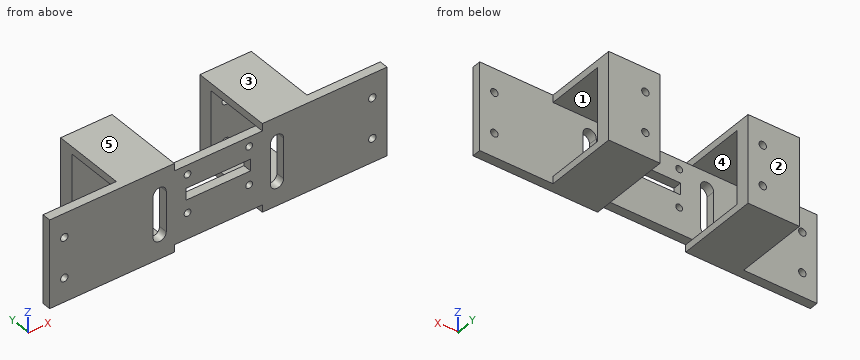
```python
from build123d import *

# Parameters (mm, degrees)
SKETCH1_W                         = 30
SKETCH1_H                         = 25
SKETCH1_R                         = 1.15
SKETCH1_W_2                       = 22
SKETCH1_H_2                       = 4
BOSS_EXTRUDE1_DEPTH               = 3
SKETCH2_W                         = 7.5
SKETCH2_H                         = 20
SKETCH2_R                         = 1.27
BOSS_EXTRUDE2_DEPTH               = 3
SKETCH6_W                         = 20
SKETCH6_H                         = 3
BOSS_EXTRUDE3_DEPTH               = 10
SKETCH7_W                         = 20
SKETCH7_H                         = 3
BOSS_EXTRUDE4_DEPTH               = 10
SKETCH8_W                         = 17.5
SKETCH8_H                         = 20
SKETCH8_R                         = 1.27
BOSS_EXTRUDE5_DEPTH               = 25
SKETCH13_W                        = 17.5
SKETCH13_H                        = 28
BOSS_EXTRUDE6_DEPTH               = 5
SKETCH14_W                        = 17.5
SKETCH14_H                        = 28
BOSS_EXTRUDE7_DEPTH               = 5
SKETCH15_W                        = 25
SKETCH15_H                        = 20
CUT_EXTRUDE2_DEPTH                = 48.5
CUT_EXTRUDE2_DEPTH_BACK           = 18.5
SKETCH16_W                        = 30
SKETCH16_H                        = 3
BOSS_EXTRUDE8_DEPTH               = 25
SKETCH19_W                        = 30
SKETCH19_H                        = 3
BOSS_EXTRUDE9_DEPTH               = 25
F_1_16_0_0625_PRESS_DOWEL_HOLE1_D = 2.54
CUT_EXTRUDE3_DEPTH                = 4


with BuildPart() as part:
    # Sketch1 → Boss-Extrude1 (new body)
    with BuildSketch(Plane(origin=(0, 0, 0), x_dir=(1, 0, 0), z_dir=(0, 1, 0))):
        with Locations((-15, 0)):
            Rectangle(SKETCH1_W, SKETCH1_H)
        with Locations((-4.5, 3.7)):
            Circle(SKETCH1_R, mode=Mode.SUBTRACT)
        with Locations((-4.5, -9.3)):
            Circle(SKETCH1_R, mode=Mode.SUBTRACT)
        with Locations((-25.5, 3.7)):
            Circle(SKETCH1_R, mode=Mode.SUBTRACT)
        with Locations((-25.5, -9.3)):
            Circle(SKETCH1_R, mode=Mode.SUBTRACT)
        with Locations((-15, -2.8)):
            Rectangle(SKETCH1_W_2, SKETCH1_H_2, mode=Mode.SUBTRACT)
    extrude(amount=BOSS_EXTRUDE1_DEPTH)

    # Sketch2 → Boss-Extrude2 (add)
    with BuildSketch(Plane(origin=(0, 3, 0), x_dir=(1, 0, 0), z_dir=(0, 1, 0))):
        with Locations((3.75, 0)):
            Rectangle(SKETCH2_W, SKETCH2_H)
        with Locations((5, 6.858)):
            Circle(SKETCH2_R, mode=Mode.SUBTRACT)
        with Locations((5, -6.858)):
            Circle(SKETCH2_R, mode=Mode.SUBTRACT)
        with Locations((-33.75, 0)):
            Rectangle(SKETCH2_W, SKETCH2_H)
        with Locations((-35, 6.858)):
            Circle(SKETCH2_R, mode=Mode.SUBTRACT)
        with Locations((-35, -6.858)):
            Circle(SKETCH2_R, mode=Mode.SUBTRACT)
    extrude(amount=-BOSS_EXTRUDE2_DEPTH)

    # Sketch6 → Boss-Extrude3 (add)
    with BuildSketch(Plane.ZY.offset(37.5)):
        with Locations((0, 1.5)):
            Rectangle(SKETCH6_W, SKETCH6_H)
    extrude(amount=BOSS_EXTRUDE3_DEPTH)

    # Sketch7 → Boss-Extrude4 (add)
    with BuildSketch(Plane(origin=(7.5, 0, 0), x_dir=(0, 0, -1), z_dir=(1, 0, 0))):
        with Locations((0, 1.5)):
            Rectangle(SKETCH7_W, SKETCH7_H)
    extrude(amount=BOSS_EXTRUDE4_DEPTH)

    # Sketch8 → Boss-Extrude5 (add)
    with BuildSketch(Plane(origin=(0, 3, 0), x_dir=(1, 0, 0), z_dir=(0, 1, 0))):
        with Locations((8.75, 0)):
            Rectangle(SKETCH8_W, SKETCH8_H)
        with Locations((5, 6.858)):
            Circle(SKETCH8_R, mode=Mode.SUBTRACT)
        with Locations((5, -6.858)):
            Circle(SKETCH8_R, mode=Mode.SUBTRACT)
        with Locations((-38.75, 0)):
            Rectangle(SKETCH8_W, SKETCH8_H)
        with Locations((-35, -6.858)):
            Circle(SKETCH8_R, mode=Mode.SUBTRACT)
        with Locations((-35, 6.858)):
            Circle(SKETCH8_R, mode=Mode.SUBTRACT)
    extrude(amount=BOSS_EXTRUDE5_DEPTH)

    # Sketch13 → Boss-Extrude6 (add)
    with BuildSketch(Plane(origin=(0, 0, -10), x_dir=(-1, 0, 0), z_dir=(0, 0, -1))):
        with Locations((38.75, 14)):
            Rectangle(SKETCH13_W, SKETCH13_H)
        with Locations((-8.75, 14)):
            Rectangle(SKETCH13_W, SKETCH13_H)
    extrude(amount=BOSS_EXTRUDE6_DEPTH)

    # Sketch14 → Boss-Extrude7 (add)
    with BuildSketch(Plane.XY.offset(10)):
        with Locations((8.75, 14)):
            Rectangle(SKETCH14_W, SKETCH14_H)
        with Locations((-38.75, 14)):
            Rectangle(SKETCH14_W, SKETCH14_H)
    extrude(amount=BOSS_EXTRUDE7_DEPTH)

    # Sketch15 → Cut-Extrude2 (cut, two sides)
    with BuildSketch(Plane(origin=(-30, 0, 0), x_dir=(0, 0, -1), z_dir=(1, 0, 0))) as cut_extrude2_sk:
        with Locations((0, 13)):
            Rectangle(SKETCH15_W, SKETCH15_H)
    extrude(amount=CUT_EXTRUDE2_DEPTH, mode=Mode.SUBTRACT)
    extrude(cut_extrude2_sk.sketch, amount=-CUT_EXTRUDE2_DEPTH_BACK, mode=Mode.SUBTRACT)

    # Sketch16 → Boss-Extrude8 (add)
    with BuildSketch(Plane.ZY.offset(47.5)):
        with Locations((0, 1.5)):
            Rectangle(SKETCH16_W, SKETCH16_H)
    extrude(amount=BOSS_EXTRUDE8_DEPTH)

    # Sketch19 → Boss-Extrude9 (add)
    with BuildSketch(Plane(origin=(17.5, 0, 0), x_dir=(0, 0, -1), z_dir=(1, 0, 0))):
        with Locations((0, 1.5)):
            Rectangle(SKETCH19_W, SKETCH19_H)
    extrude(amount=BOSS_EXTRUDE9_DEPTH)

    # 1/16 (0.0625) Press Dowel Hole1 (through all)
    with Locations(Plane(origin=(0, 3, 0), x_dir=(1, 0, 0), z_dir=(0, 1, 0))):
        with Locations((-67.5, 6.858), (-67.5, -6.858), (37.5, -6.858), (37.5, 6.858)):
            Hole(F_1_16_0_0625_PRESS_DOWEL_HOLE1_D / 2)

    # Sketch21 → Cut-Extrude3 (cut, through all)
    with BuildSketch(Plane(origin=(0, 3, 0), x_dir=(1, 0, 0), z_dir=(0, 1, 0))):
        with BuildLine():
            Line((2.75, -6.858), (2.75, 6.858))
            ThreePointArc((2.75, 6.858), (5, 9.108), (7.25, 6.858))
            Line((7.25, 6.858), (7.25, -6.858))
            ThreePointArc((7.25, -6.858), (5, -9.108), (2.75, -6.858))
        make_face()
        with BuildLine():
            Line((-32.75, 6.858), (-32.75, -6.858))
            ThreePointArc((-32.75, -6.858), (-35, -9.108), (-37.25, -6.858))
            Line((-37.25, -6.858), (-37.25, 6.858))
            ThreePointArc((-37.25, 6.858), (-35, 9.108), (-32.75, 6.858))
        make_face()
    extrude(amount=-CUT_EXTRUDE3_DEPTH, mode=Mode.SUBTRACT)


solid = part.part
```
Check sheet for the modelled part. Datum: model origin and axes. Units: mm. Face numbers are marked on the shaded views. A direction names the side the tool comes from. Round coordinates to 2 decimals unless told otherwise and drop trailing zeros. Order: outer loops, then holes, each group sorted by start corner. A loop starts at its lowest first (then second) coordinate and runs counter-clockwise, first axis right, second up. Notation, with made-up numbers: (-16, 84) -> (11, 84) arc R22 cw to (11, 106) -> close; hole circle Ø8 at (-33, 25.5). An arc over 180 degrees is marked (long way). One line per item, written item: value. Start each with the question number.
Q1. Mould release check, pull along Z, two halves, no side actions. Record for the marked faces 1, 2 and 3: pulls with the +Z half, pulls with the -Z half, needs draft (parallel to the pull), parting line crosses it, or undercut.
Q2. Thickness scan on line 1 (Z direction, x = -25.5, y = 2.1); line 2 (Z direction, x = 5, y = 25.05); line 3 (X direction, y = 0.95, z = -3.7). Record the ranges inside material, lowest first.
Q3. Cross-section at C-C (z = -3.7). Record the boundary of the cut face in (x, y), and give its area (3 significant figures).
Q4. Gauge pin test, flat ends, axial feed: pin 1 Ø3.5 at (x, y) = (-16, 1) entering from +Z; pin 2 Ø2 at (x, z) = (-25.5, -3.7) entering from +Y; pin 3 Ø2.5 at (x, z) = (-4.5, -3.7) entering from -Y; pin 4 Ø14 at (y, z) = (19, -3.5) entering from -X. Record the tip position at first contact, or that the pin passes through.
Q5. Cross-section at B-B (x = -67.5). Record the boundary of the cut face in (y, z).
Q6. Cross-section at D-D (x = -14.5). Record the boundary of the cut face in (y, z), and give its area (3 significant figures).
Q7. Cross-section at A-A (y = 25). Record the boundary of the cut face in (x, z), and give its area (3 significant figures).
Q8. Set-up check for the marked faces 4 and 5: record each of +Z, -Z, +X, -X, +Y, -Y from which the full face is reachable in a straight line by a thin tool's end or side.
Completed:
1. face 1: undercut
1. face 2: needs draft
1. face 3: pulls with the +Z half
2. line 1: z = -12.5 to -4.85, -2.55 to 0.8, 4.8 to 8.15, 10.45 to 12.5
2. line 2: z = -15 to -8.13, -5.59 to 5.59, 8.13 to 15
2. line 3: x = -72.5 to -37.25, -32.75 to -26.65, -24.35 to -5.65, -3.35 to 2.75, 7.25 to 42.5
3. outline: (-72.5, 0) -> (-37.25, 0) -> (-37.25, 3) -> (-72.5, 3) -> close; (-47.5, 23) -> (-30, 23) -> (-30, 28) -> (-47.5, 28) -> close; (-32.75, 0) -> (-26.65, 0) -> (-26.65, 3) -> (-32.75, 3) -> close; (-24.35, 0) -> (-5.65, 0) -> (-5.65, 3) -> (-24.35, 3) -> close; (-3.35, 0) -> (2.75, 0) -> (2.75, 3) -> (-3.35, 3) -> close; (0, 23) -> (17.5, 23) -> (17.5, 28) -> (0, 28) -> close; (7.25, 0) -> (42.5, 0) -> (42.5, 3) -> (7.25, 3) -> close
3. area: 479 mm²
4. pin 1: stops at z = 12.5
4. pin 2: passes through
4. pin 3: stops at y = 0
4. pin 4: stops at x = -47.5
5. outline: (0, -15) -> (3, -15) -> (3, -8.13) -> (0, -8.13) -> close; (0, -5.59) -> (3, -5.59) -> (3, 5.59) -> (0, 5.59) -> close; (0, 8.13) -> (3, 8.13) -> (3, 15) -> (0, 15) -> close
6. outline: (0, -12.5) -> (3, -12.5) -> (3, 0.8) -> (0, 0.8) -> close; (0, 4.8) -> (3, 4.8) -> (3, 12.5) -> (0, 12.5) -> close
6. area: 63.0 mm²
7. outline: (-47.5, -15) -> (-30, -15) -> (-30, 15) -> (-47.5, 15) -> close; (0, -15) -> (17.5, -15) -> (17.5, 15) -> (0, 15) -> close; hole circle Ø2.54 at (-35, -6.86); hole circle Ø2.54 at (-35, 6.86); hole circle Ø2.54 at (5, -6.86); hole circle Ø2.54 at (5, 6.86)
7. area: 1,030 mm²
8. face 4: +X, -X
8. face 5: +Z, +X, -X, +Y, -Y
